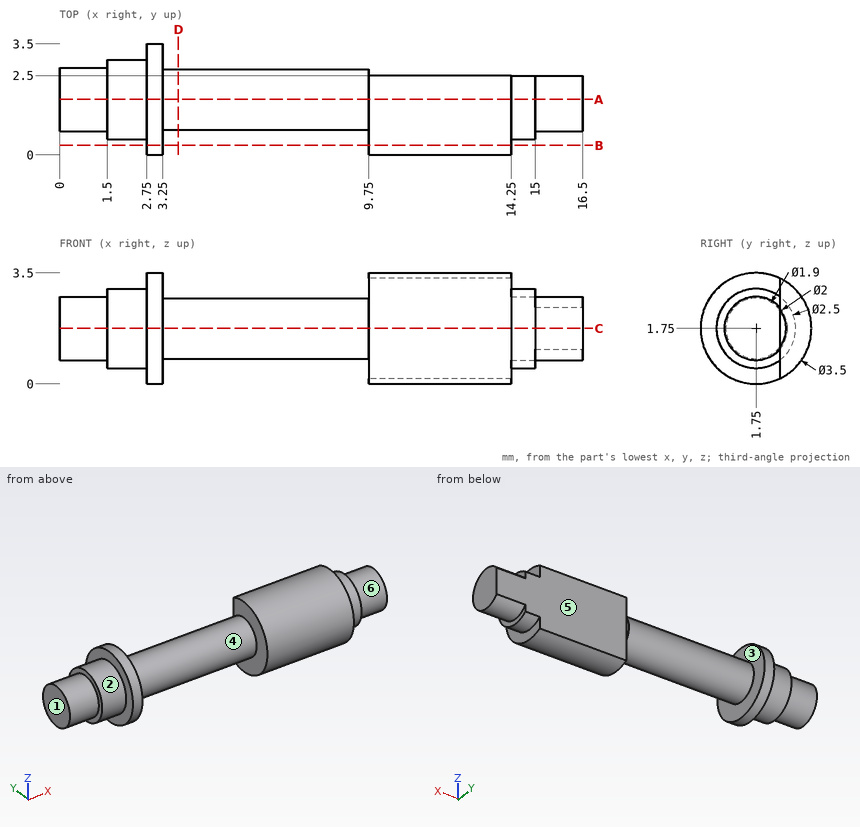
Job drawing, mm, ordinate dimensions from the low corner. One solid piece. A direction names the side the tool comes from. Give positions to 0.01 mm unless a question says otherwise; leave off trailing zeros. Loops run counter-clockwise (first coordinate to the right, second up) from the corner with the lowest first, then second, coordinate; pieces in that order, holes last.
Item 1: Which spindle directions (+Z, -Z, +X, -X, +Y, -Y) get a long thin tool onto all of the face, cutting with end or side? Do the marked faces 4, 5 and 6. Say none if no direction does.
Answers follow:
face 4: none
face 5: +Z, -Z, +X, +Y
face 6: +X
Item 2: Slice it at C-C, the plane z = 1.75. List the corners of the cut face in (x, y), and give its area (3 significant figures).
Answers follow:
outline: (0, 0.75) - (1.5, 0.75) - (1.5, 0.5) - (2.75, 0.5) - (2.75, 0) - (3.25, 0) - (3.25, 0.8) - (9.75, 0.8) - (9.75, 0) - (14.25, 0) - (14.25, 0.5) - (15, 0.5) - (15, 0.75) - (16.5, 0.75) - (16.5, 2.5) - (9.75, 2.5) - (9.75, 2.7) - (3.25, 2.7) - (3.25, 3.5) - (2.75, 3.5) - (2.75, 3) - (1.5, 3) - (1.5, 2.75) - (0, 2.75) - close
area: 35.6 mm2
Item 3: Flat gauge pin, fed straight in: pin 1 (1 mm diameter, centred on x = 11, z = 1.5, fed in from +Y). Where does the tip first touch, or does it go through?
Answers follow:
pin 1: stops at y = 2.5
Item 4: Slice it at D-D, the plane x = 3.75. List the corners of the cut face in (y, z).
Answers follow:
outline: circle Ø1.9 at (1.75, 1.75)
Item 5: Drill centre lines: line 1 (X direction, y = 1.4, z = 0.35); line 2 (X direction, y = 2.25, z = 0.65); line 3 (Y direction, x = 12.5, z = 1.75). Where is each one in solid material? Low to high.
Answers follow:
line 1: x = 2.75 to 3.25, 9.75 to 14.25
line 2: x = 1.5 to 3.25, 9.75 to 15
line 3: y = 0 to 2.5
Item 6: Pull direction X, two halves, no side cores. Call the marked faces 1, 2 and 3: released by +X, released by -X, zero draft, split by the parting line, or undercut.
Answers follow:
face 1: released by -X
face 2: zero draft
face 3: undercut
Item 7: Slice it at B-B, the plane y = 0.3. List the corners of the cut face in (x, z).
Answers follow:
outline: (2.75, 0.77) - (3.25, 0.77) - (3.25, 2.73) - (2.75, 2.73) - close; (9.75, 0.77) - (14.25, 0.77) - (14.25, 2.73) - (9.75, 2.73) - close
Item 8: Slice it at A-A, the plane y = 1.75. List the corners of the cut face in (x, z), and give its area (4 significant figures).
Answers follow:
outline: (0, 0.75) - (1.5, 0.75) - (1.5, 0.5) - (2.75, 0.5) - (2.75, 0) - (3.25, 0) - (3.25, 0.8) - (9.75, 0.8) - (9.75, 0) - (14.25, 0) - (14.25, 0.5) - (15, 0.5) - (15, 0.75) - (16.5, 0.75) - (16.5, 2.75) - (15, 2.75) - (15, 3) - (14.25, 3) - (14.25, 3.5) - (9.75, 3.5) - (9.75, 2.7) - (3.25, 2.7) - (3.25, 3.5) - (2.75, 3.5) - (2.75, 3) - (1.5, 3) - (1.5, 2.75) - (0, 2.75) - close
area: 40.85 mm2
